Input: part model. Units: mm. Frame: model coordinates. A direction names the side the tool comes from. Coordinates: 2 decimals unless noted, no trailing zeros. Loops run counter-clockwise (first coordinate to the right, second up) from the corner with the lowest first, then second, coordinate; pieces in that order, holes last. Notation, with made-up numbers: (-36, 47.5) - (-6, 47.5) arc R25 ccw to (-6, 59.5) - close; hole circle Ø6 at (5, 2.5). An arc over 180 degrees is marked (long way). Use one line per item in the form item = value.
from build123d import *

# Parameters (mm, degrees)
SKETCH2_R           = 14
SKETCH2_R_2         = 19
SKETCH2_R_3         = 6
BOSS_EXTRUDE1_DEPTH = 12
FILLET1_R           = 38


with BuildPart() as part:
    # Sketch2 → Boss-Extrude1 (new body)
    # profile 1 of 3: a face of its own
    with BuildSketch(Plane(origin=(0, 0, 0), x_dir=(1, 0, 0), z_dir=(0, 1, 0))):
        with BuildLine():
            Line((31, 0), (18.395196505, 48.755706629))
            ThreePointArc((18.395196505, 48.755706629), (18.848192667, 46.397005048), (19, 44))
            ThreePointArc((19, 44), (-2.397005048, 25.151807333), (-18.395196505, 48.755706629))
            Line((-18.395196505, 48.755706629), (-31, 0))
            Line((-31, 0), (-18.395196505, -48.755706629))
            ThreePointArc((-18.395196505, -48.755706629), (-2.397005048, -25.151807333), (19, -44))
            ThreePointArc((19, -44), (18.848192667, -46.397005048), (18.395196505, -48.755706629))
            Line((18.395196505, -48.755706629), (31, 0))
        make_face()
        with Locations(Location((0, 0, 0), (0, 0, 270))):
            Circle(SKETCH2_R, mode=Mode.SUBTRACT)
    # profile 2 of 3: a face of its own
    with BuildSketch(Plane(origin=(0, 0, 0), x_dir=(1, 0, 0), z_dir=(0, 1, 0))):
        with Locations((0, -44)):
            Circle(SKETCH2_R_2)
        with Locations(Location((0, -44, 0), (0, 0, 270))):
            Circle(SKETCH2_R_3, mode=Mode.SUBTRACT)
    # profile 3 of 3: a face of its own
    with BuildSketch(Plane(origin=(0, 0, 0), x_dir=(1, 0, 0), z_dir=(0, 1, 0))):
        with Locations((0, 44)):
            Circle(SKETCH2_R_2)
        with Locations(Location((0, 44, 0), (0, 0, 270))):
            Circle(SKETCH2_R_3, mode=Mode.SUBTRACT)
    extrude(amount=BOSS_EXTRUDE1_DEPTH)

    # Fillet1
    fillet1_edges = [part.edges().sort_by_distance(p)[0] for p in [
        (-31, 6, 0),
        (31, 6, 0),
    ]]
    fillet(fillet1_edges, radius=FILLET1_R)

    # Sketch3 → Revolve1 (revolve)
    with BuildSketch(Plane.XY, mode=Mode.PRIVATE) as revolve1_sk:
        Polygon((14, 0), (28, 0), (28, -30), (14, -21.917096231), align=None)
    revolve(revolve1_sk.sketch.rotate(Axis((0, 0, 0), (0, -1, 0)), 90), axis=Axis((0, 0, 0), (0, -1, 0)))


solid = part.part
Q1. Cut plane B-B, the plane z = 0. Return loops of the section in (x, y), then the cut area to 3 significant figures.
Check values:
outline = (-29.75, 0) - (-28, 0) - (-28, -30) - (-14, -21.92) - (-14, 12) - (-29.75, 12) - close; (14, -21.92) - (28, -30) - (28, 0) - (29.75, 0) - (29.75, 12) - (14, 12) - close
area = 1,100 mm²
Q2. Cut plane C-C, the plane x = 0. Return loops of the section in (y, z).
Check values:
outline = (-30, -28) - (0, -28) - (0, -38) - (12, -38) - (12, -14) - (-21.92, -14) - close; (-30, 28) - (-21.92, 14) - (12, 14) - (12, 38) - (0, 38) - (0, 28) - close; (0, -63) - (12, -63) - (12, -50) - (0, -50) - close; (0, 50) - (12, 50) - (12, 63) - (0, 63) - close
Q3. Pull-direction query (Z, two-part tool) for faces 3 (the cylindrical face through (0, 6, 38)), 4 (the flat face through (-23.54, 5.92, 28.86)), 5 (the flat face through (0, 12, -15)); classes: pulls with the +Z half, pulls with the -Z half, needs draft (parallel to the pull), parting line crosses it, or undercut.
Check values:
face_3 = undercut
face_4 = pulls with the +Z half
face_5 = needs draft
Q4. Cut plane D-D, the plane y = -18. Return loops of the section in (x, z).
Check values:
outline = circle Ø56 at (0, 0); hole circle Ø28 at (0, 0)
Q5. Set-up query: faces 1 (the cylindrical face through (12.4, -4.7, 6.5)), 2 (the cylindrical face through (24.84, -15.21, 12.92)). Return all of +Z, -Z, +X, -X, +Y, -Y with unobstructed straight access to the full face (end or side cutting, diameter ignored); none if empty.
Check values:
face_1 = +Y, -Y
face_2 = -Y
Q6. First-contact query: P1, Ø1.5, axis at x = 13.5, y = 3.5, coming from the +Z side; P2, Ø2, axis at y = 6.5, z = 11, coming from the +X side; P3, Ø3, axis at x = -21.5, z = 3, coming from the -Y side. Flat tips, straight axial feed; report the tip coordinate or a pass-through.
Check values:
P1 = 58.09
P2 = 28.41
P3 = -27.23
Q7. Ray query, line 1 along Z through (x, y) = (2, 2.5); line 2 along X through (y, z) = (-11, 0); line 3 along X through (y, z) = (2.5, -44). Return the intervals inside material, ascending. Write a range as [from, to].
Check values:
line_1 = [-62.89, -49.66], [-38.34, -13.86], [13.86, 38.34], [49.66, 62.89]
line_2 = [-28, -14], [14, 28]
line_3 = [-19.62, -6], [6, 19.62]
Q8. Cut plane A-A, the plane y = 2.5. Return loops of the section in (x, z).
Check values:
outline = (-28.54, -9.51) - (-18.4, -48.76) arc R19 ccw to (18.4, -48.76) - (28.54, -9.51) arc R38 ccw to (28.54, 9.51) - (18.4, 48.76) arc R19 ccw to (-18.4, 48.76) - (-28.54, 9.51) arc R38 ccw to start; hole circle Ø28 at (0, 0); hole circle Ø12 at (0, -44); hole circle Ø12 at (0, 44)
